The model under review builds one solid part; all positions refer to its coordinate system, in mm. Face numbers are marked on the shaded views. Coordinates: 2 decimals unless noted, no trailing zeros. Write each loop counter-clockwise with the first axis right and the second up, starting at its lowest first coordinate (ties: lowest second). Pieces come first, ordered by that corner, then holes. Notation, with made-up numbers: M 73,5 L 88,5 A15 ccw 88,15 Z; hole C 14,-22.75 d9. An arc over 180 degrees is marked long. Answer as a JSON object with one key per item and string values.
```python
from build123d import *

# Parameters (mm, degrees)
SKETCH2_R               = 50
BOSS_EXTRUDE1_DEPTH     = 23.5
SKETCH3_R               = 47
CUT_EXTRUDE1_DEPTH      = 20.5
BOSS_EXTRUDE2_DEPTH     = 20.5
SKETCH7_R               = 1.5
CUT_EXTRUDE3_DEPTH      = 12
SKETCH8_R               = 3.1
CUT_EXTRUDE4_DEPTH      = 75.51342161
CUT_EXTRUDE5_REACH      = 78.559
CUT_EXTRUDE5_END_RADIUS = 47
CUT_EXTRUDE6_DEPTH      = 75.513421776


with BuildPart() as part:
    # Sketch2 → Boss-Extrude1 (new body)
    with BuildSketch(Plane(origin=(0, 0, 0), x_dir=(1, 0, 0), z_dir=(0, 1, 0))):
        with Locations(Location((0, 0, 0), (0, 0, 270))):
            Circle(SKETCH2_R)
    extrude(amount=BOSS_EXTRUDE1_DEPTH)

    # Sketch3 → Cut-Extrude1 (cut)
    with BuildSketch(Plane(origin=(0, 23.5, 0), x_dir=(1, 0, 0), z_dir=(0, 1, 0))):
        with Locations(Location((0, 0, 0), (0, 0, 270))):
            Circle(SKETCH3_R)
    extrude(amount=-CUT_EXTRUDE1_DEPTH, mode=Mode.SUBTRACT)

    # Sketch4 → Boss-Extrude2 (add)
    with BuildSketch(Plane(origin=(0, 3, 0), x_dir=(1, 0, 0), z_dir=(0, 1, 0))):
        with BuildLine():
            Line((3, 48.95), (-3, 48.95))
            Line((-3, 48.95), (-3, 45.95))
            ThreePointArc((-3, 45.95), (0, 42.95), (3, 45.95))
            Line((3, 45.95), (3, 48.95))
        make_face()
        with BuildLine():
            Line((43.891943515, -21.876923789), (41.293867304, -20.376923789))
            ThreePointArc((41.293867304, -20.376923789), (37.195791093, -21.475), (38.293867304, -25.573076211))
            Line((38.293867304, -25.573076211), (40.891943515, -27.073076211))
            Line((40.891943515, -27.073076211), (43.891943515, -21.876923789))
        make_face()
        with BuildLine():
            Line((-40.891943515, -27.073076211), (-38.293867304, -25.573076211))
            ThreePointArc((-38.293867304, -25.573076211), (-37.195791093, -21.475), (-41.293867304, -20.376923789))
            Line((-41.293867304, -20.376923789), (-43.891943515, -21.876923789))
            Line((-43.891943515, -21.876923789), (-40.891943515, -27.073076211))
        make_face()
    extrude(amount=BOSS_EXTRUDE2_DEPTH)

    # Sketch7 → Cut-Extrude3 (cut)
    with BuildSketch(Plane(origin=(0, 23.5, 0), x_dir=(1, 0, 0), z_dir=(0, 1, 0))):
        with Locations(Location((0, 45.95, 0), (0, 0, 270))):
            Circle(SKETCH7_R)
        with Locations(Location((39.793867304, -22.975, 0), (0, 0, 270))):
            Circle(SKETCH7_R)
        with Locations(Location((-39.793867304, -22.975, 0), (0, 0, 270))):
            Circle(SKETCH7_R)
    extrude(amount=-CUT_EXTRUDE3_DEPTH, mode=Mode.SUBTRACT)

    # Sketch8 → Cut-Extrude4 (cut, through all)
    with BuildSketch(Plane.XY):
        with Locations(Location((0, 7.6, 0), (0, 0, 180))):
            Circle(SKETCH8_R)
    extrude(amount=CUT_EXTRUDE4_DEPTH, mode=Mode.SUBTRACT)

    # Cut-Extrude5: up to this cylinder (the profile starts inside it)
    cut_extrude5_end = Plane(origin=(0, 10.013188, 0), z_dir=(0, 1, 0)) * Cylinder(CUT_EXTRUDE5_END_RADIUS, 252.118, mode=Mode.PRIVATE)
    # Sketch9 → Cut-Extrude5 (cut, up to the surface)
    with BuildSketch(Plane(origin=(3, 0, 0), x_dir=(0, 0, -1), z_dir=(1, 0, 0)), mode=Mode.PRIVATE) as cut_extrude5_sk1:
        Polygon((46.904157598, 12.941577654), (42.581578264, 20.428504681), (42.581578264, 3), (46.904157598, 3), align=None)
    cut_extrude5_tool1 = extrude(cut_extrude5_sk1.sketch, amount=-CUT_EXTRUDE5_REACH, mode=Mode.PRIVATE) & cut_extrude5_end
    add(cut_extrude5_tool1.solids().sort_by_distance((3, 10.013188, -44.545799))[0], mode=Mode.SUBTRACT)

    # Sketch11 → Cut-Extrude6 (cut, through all)
    with BuildSketch(Plane.XY):
        with BuildLine():
            Line((-2.5, 9.5), (2.5, 9.5))
            ThreePointArc((2.5, 9.5), (5.5, 6.5), (2.5, 3.5))
            Line((2.5, 3.5), (-2.5, 3.5))
            ThreePointArc((-2.5, 3.5), (-5.5, 6.5), (-2.5, 9.5))
        make_face()
    extrude(amount=-CUT_EXTRUDE6_DEPTH, mode=Mode.SUBTRACT)


solid = part.part
```
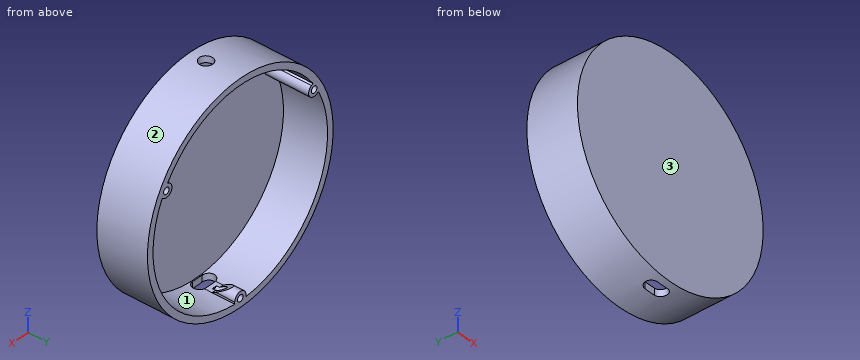
(1) Add section D-D on x = 32.5. Give the boundary of the cut face in (y, z).
Results list:
{"outline": "M 0,-38 L 23.5,-38 L 23.5,-33.95 L 3,-33.95 L 3,33.95 L 23.5,33.95 L 23.5,38 L 0,38 Z"}
(2) For pin 1 Ø1.5 at (x, z) = (-18.5, -13.5) entering from +Y; pin 2 Ø0.6 at (x, y) = (-1, 3.5) entering from +Z; pin 3 Ø4 at (y, z) = (19, -26.5) entering from +X; pin 4 Ø3.5 at (x, y) = (0, 7.6) entering from -Z, all flat-tipped, find the tip position at first contact; note any pin that passes through.
Results list:
{"pin 1": "y = 3", "pin 2": "z = 50", "pin 3": "x = 43.59", "pin 4": "through"}
(3) Draft analysis for pull direction X (two halves, no side actions). For the marked faces 1, 2 and 3, state which applies: released by +X, released by -X, zero draft, split by the parting line, or undercut.
Results list:
{"face 1": "undercut", "face 2": "split by the parting line", "face 3": "zero draft"}
(4) Add section B-B on y = 16. Give the boundary of the cut face in (x, z) (3 decimals), and give its area (3 significant figures).
Results list:
{"outline": "C 0,0 d100; hole M -42.12,20.854 A47 ccw -3,-46.904 L -3,-45.95 A3 cw -2.888,-45.138 L -1.261,-45.138 A1.5 ccw long 1.261,-45.138 L 2.888,-45.138 A3 cw 3,-45.95 L 3,-46.904 A47 ccw 42.12,20.854 L 41.294,20.377 A3 cw 38.294,25.573 L 39.12,26.05 A47 ccw -39.12,26.05 L -38.294,25.573 A3 cw -41.294,20.377 Z; hole C -39.794,22.975 d3; hole C 39.794,22.975 d3", "area": "946 mm²"}
(5) Add section A-A on x = 0. Give the boundary of the cut face in (y, z), and give its area (3 significant figures).
Results list:
{"outline": "M 0,-50 L 3.5,-50 L 3.5,-46.9 L 3,-46.9 L 3,47 L 4.5,47 L 4.5,50 L 0,50 Z; M 9.5,-50 L 23.5,-50 L 23.5,-47.45 L 11.5,-47.45 L 11.5,-46.9 L 9.5,-46.9 Z; M 10.7,47 L 23.5,47 L 23.5,50 L 10.7,50 Z; M 17.19,-44.45 L 23.5,-44.45 L 23.5,-42.95 L 19.79,-42.95 Z", "area": "389 mm²"}
(6) Wall thickness on line 1 along Y through (x, z) = (28.5, 10); line 2 along Y through (x, z) = (0, 47.75); line 3 along Z through (x, y) = (32.5, 15.75): over which ranges is each line inside the solid? List them lowest first. Write a range as from..to.
Results list:
{"line 1": "0..3", "line 2": "0..4.5, 10.7..23.5", "line 3": "-38..-33.95, 33.95..38"}
(7) Add section C-C on z = 7. Give the boundary of the cut face in (x, y), and give its area (3 significant figures).
Results list:
{"outline": "M -49.51,0 L 49.51,0 L 49.51,23.5 L 46.48,23.5 L 46.48,3 L -46.48,3 L -46.48,23.5 L -49.51,23.5 Z", "area": "421 mm²"}
